Answer from the drawing. Dimensions are ordinates in mm from the lowest x, y and z of the part. Coordinates: 2 decimals unless noted, no trailing zeros. Write each loop counter-clockwise with the first axis right and the second up, starting at its lowest first coordinate (ties: lowest second). Pieces come first, ordered by that corner, then holes. Notation, with made-up numbers: (-3, 88.5) -> (40, 88.5) arc R20 ccw to (40, 118.5) -> close; hole circle Ø9 at (37, 72.5). An arc over 180 degrees is marked (long way). One line per item, written item: value. Start each with the question number.
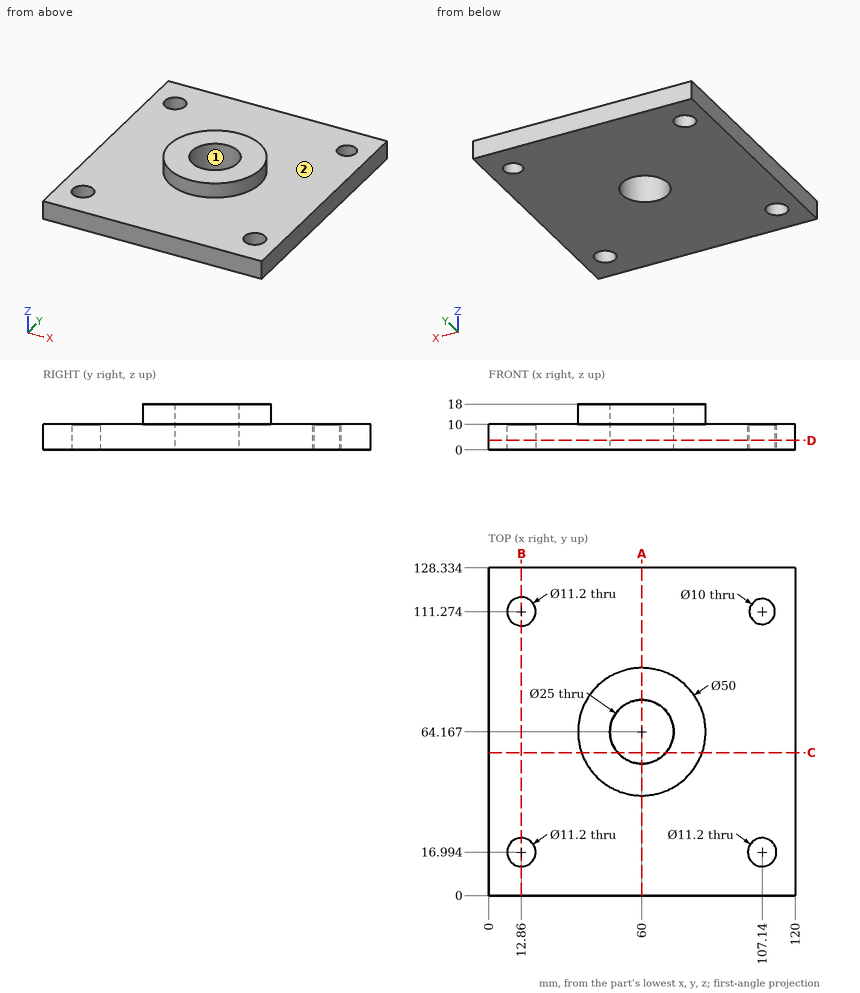
1. A cutting plane is placed at D-D on z = 3.75. Give the vertices of the cut face in (x, y), then the cut area to 3 significant figures.
2. Find the intervals of material crossed by probe 1 along Y at (x, z) = (107.14, 3.5); probe 2 along Y at (x, z) = (12.86, 3.5); probe 3 along X at (y, z) = (13.5, 9.5), in increasing order. Write a range as from..to.
3. For a pull along X with two mould halves and no side action, classify the marked faces 1 and 2 as +X half, -X half, draft (parallel to the pull), parting line (faces both ways), or undercut.
4. A cutting plane is placed at B-B on x = 12.86. Give the vertices of the cut face in (y, z).
5. A cutting plane is placed at A-A on x = 60. Give the vertices of the cut face in (y, z), then the cut area to 3 significant figures.
6. Given pin 1 (13 mm diameter, centred on x = 12.86, y = 16.99, fed in from -Z); pin 2 (6 mm diameter, centred on x = 107.14, y = 111.27, fed in from +Z); pin 3 (6 mm diameter, centred on x = 21.5, y = 95.5, fed in from +Z), each flat-ended and moving along its own axis, determine where each tip first touches the part or whether it passes through.
7. A cutting plane is placed at C-C on y = 56. Give the vertices of the cut face in (x, z).
Derived:
1. outline: (0, 0) -> (120, 0) -> (120, 128.33) -> (0, 128.33) -> close; hole circle Ø11.2 at (12.86, 16.99); hole circle Ø11.2 at (12.86, 111.27); hole circle Ø25 at (60, 64.17); hole circle Ø11.2 at (107.14, 16.99); hole circle Ø10 at (107.14, 111.27)
1. area: 14,500 mm2
2. probe 1: y = 0..11.39, 22.59..106.27, 116.27..128.33
2. probe 2: y = 0..11.39, 22.59..105.67, 116.87..128.33
2. probe 3: x = 0..8.48, 17.24..102.76, 111.52..120
3. face 1: undercut
3. face 2: draft
4. outline: (0, 0) -> (11.39, 0) -> (11.39, 10) -> (0, 10) -> close; (22.59, 0) -> (105.67, 0) -> (105.67, 10) -> (22.59, 10) -> close; (116.87, 0) -> (128.33, 0) -> (128.33, 10) -> (116.87, 10) -> close
5. outline: (0, 0) -> (51.67, 0) -> (51.67, 18) -> (39.17, 18) -> (39.17, 10) -> (0, 10) -> close; (76.67, 0) -> (128.33, 0) -> (128.33, 10) -> (89.17, 10) -> (89.17, 18) -> (76.67, 18) -> close
5. area: 1,230 mm2
6. pin 1: stops at z = 0
6. pin 2: passes through
6. pin 3: stops at z = 10
7. outline: (0, 0) -> (50.54, 0) -> (50.54, 18) -> (36.37, 18) -> (36.37, 10) -> (0, 10) -> close; (69.46, 0) -> (120, 0) -> (120, 10) -> (83.63, 10) -> (83.63, 18) -> (69.46, 18) -> close
